Autodesk Inventor part; units mm, degrees
ref_plane "YZ Plane" through (0, 0, 0) normal (1, 0, 0) x (0, 1, 0)
ref_plane "XZ Plane" through (0, 0, 0) normal (0, 1, 0) x (-1, 0, 0)
ref_plane "XY Plane" through (0, 0, 0) normal (0, 0, 1) x (1, 0, 0)
sketch "Sketch1" plane through (0, 0, 0) normal (0, 1, 0) x (-1, 0, 0)
  line L0 (0, 0) -> (-400, 0)
  line L1 (-400, 0) -> (-400, -300)
  line L2 (-400, -300) -> (0, -300)
  line L3 (0, -300) -> (0, 0)
  line L4 (0, -200) -> (-400, -200)
  line L5 (0, -100) -> (-400, -100)
  dimension "d0" = 400
  dimension "d1" = 300
  dimension "d21" = 100
  dimension "d22" = 100
extrude "Extrusion1" add sketch "Sketch1" along normal blind 10 contours L3 L2 L1 L4
extrude "Extrusion2" add sketch "Sketch1" along normal blind 35 contours L3 L4 L1 L5
extrude "Extrusion3" add sketch "Sketch1" along normal blind 60 contours L3 L5 L1 L0
sketch "Sketch2" plane through (0, 60, 0) normal (0, 1, 0) x (1, 0, 0)
  line L0 (0, 300) -> (0, 0)
  line L1 (0, 50) -> (400, 50) construction
  line L2 (400, 0) -> (400, 300)
  line L3 (0, 0) -> (400, 0)
  line L4 (0, 100) -> (0, 0)
  circle A0 centre (100, 50) radius 5
  circle A1 centre (200, 50) radius 5
  circle A2 centre (300, 50) radius 5
  point P0 (0, 50)
  dimension "d30" = 50
  dimension "d32" = 100
  dimension "d33" = 100
  dimension "d34" = 100
  dimension "d35" = 10
  dimension "d36" = 10
  dimension "d37" = 10
extrude "Extrusion4" add sketch "Sketch2" along normal blind 110
chamfer "Chamfer1" distance 4 angle 45 3 edges at (295, 170, -50) (195, 170, -50) (95, 170, -50)
sketch "Sketch3" plane through (0, 35, 0) normal (0, 1, 0) x (1, 0, 0)
  line L0 (0, 200) -> (0, 100)
  line L1 (0, 150) -> (400, 150) construction
  line L2 (400, 0) -> (400, 300)
  circle A0 centre (100, 150) radius 5
  circle A1 centre (200, 150) radius 5
  circle A2 centre (300, 150) radius 5
  point P0 (0, 0)
  dimension "d43" = 100
  dimension "d44" = 100
  dimension "d45" = 100
  dimension "d46" = 10
  dimension "d47" = 10
  dimension "d48" = 10
extrude "Extrusion5" add sketch "Sketch3" along normal blind 25
sketch "Sketch4" plane through (0, 10, 0) normal (0, 1, 0) x (1, 0, 0)
  line L0 (0, 300) -> (0, 200)
  line L1 (0, 250) -> (400, 250) construction
  line L2 (400, 0) -> (400, 300)
  circle A0 centre (133.3333, 250) radius 5
  circle A1 centre (266.6667, 250) radius 5
  point P0 (0, 0)
  dimension "d51" = 133.3333
  dimension "d52" = 133.3333
  dimension "d53" = 10
  dimension "d54" = 10
extrude "Extrusion6" add sketch "Sketch4" along normal blind 25
chamfer "Chamfer2" distance 4 angle 45 5 edges at (295, 60, -150) (261.6667, 35, -250) (128.3333, 35, -250) (95, 60, -150) (195, 60, -150)
chamfer "Chamfer3" distance 6.5 angle 61.2 1 edges at (295, 60, -50) measured on face at (200.2009, 60, -84.9878)
chamfer "Chamfer4" distance 6.5 angle 61.2 2 edges at (195, 60, -50) (95, 60, -50) measured on face at (200.2009, 60, -84.9878)
chamfer "Chamfer5" distance 6.5 angle 61.2 3 edges at (295, 35, -150) (195, 35, -150) (95, 35, -150) measured on face at (200.2009, 35, -184.9878)
chamfer "Chamfer6" distance 6.5 angle 61.2 2 edges at (128.3333, 10, -250) (261.6667, 10, -250) measured on face at (222.0213, 10, -215.0122)
The listing builds one solid part. Answer for the finished solid, in the listing's coordinates (mm). A direction names the side the tool comes from. Round coordinates to 2 decimals unless told otherwise and drop trailing zeros. Loops run counter-clockwise (first coordinate to the right, second up) from the corner with the lowest first, then second, coordinate; pieces in that order, holes last.
Q1. Which of the six approach directions +Z, -Z, +X, -X, +Y, -Y give full straight-line access (tool end or side, diameter ignored) to faces 4 (the face through (269.35, 26.35, -245.78)), 5 (the face through (197, 47, -100)), 6 (the face through (400, 23, -115))?
Q2. Given pin 1 Ø6 at (x, z) = (298.5, -268.5) entering from +Y; pin 2 Ø20 at (x, y) = (136.5, 23) entering from -Z; pin 3 Ø0.6 at (x, z) = (133.5, -250) entering from +Y, each flat-ended and moving along its own axis, determine where each tip first touches the part or whether it passes through.
Q3. For a pull along Z with two mould halves and no side action, classify faces 1 (the face through (95.48, 69.77, -45.86)), 2 (the face through (203, 60, -38)), 3 (the face through (104.619, 51.347, -151.915)) as released by +Z, released by -Z, zero draft, split by the parting line, or undercut.
Q4. Section B-B, the plane y = 97.5 is taken. Determine the outline of the cut face in (x, z).
Q5. Find the intervals of material crossed by line 1 (Z direction, x = 307, y = 27.5); line 2 (Y direction, x = 376, z = -103.5); line 3 (Z direction, x = 171.5, y = 39), in increasing order.
Q6. Section A-A, the plane x = 345.5 is taken. Determine the outline of the cut face in (y, z).
Q7. Section C-C, the plane z = -128.5 is taken. Determine the outline of the cut face in (x, y), then the cut area to 3 significant figures.
Completed:
1. face 4: +Y
1. face 5: +X, -X, +Y
1. face 6: +Z, -Z, +X, +Y, -Y
2. pin 1: stops at y = 10
2. pin 2: stops at z = -259.67
2. pin 3: stops at y = 35
3. face 1: split by the parting line
3. face 2: zero draft
3. face 3: undercut
4. outline: circle Ø10 at (100, -50); circle Ø10 at (200, -50); circle Ø10 at (300, -50)
5. line 1: z = -200 to 0
5. line 2: y = 0 to 35
5. line 3: z = -100 to 0
6. outline: (0, -300) - (10, -300) - (10, -200) - (35, -200) - (35, -100) - (60, -100) - (60, 0) - (0, 0) - close
7. outline: (0, 0) - (400, 0) - (400, 35) - (0, 35) - close
7. area: 14,000 mm2
